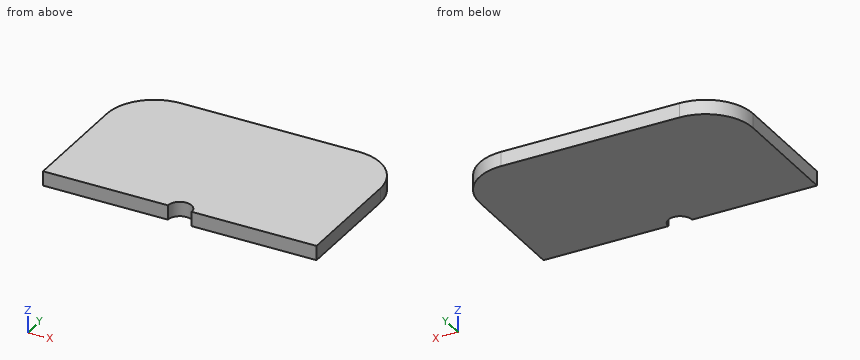
```python
from build123d import *

# Parameters (mm, degrees)
PAD_DEPTH = 15.45


with BuildPart() as part:
    # Sketch → Pad (new body)
    with BuildSketch(Plane.XY):
        with BuildLine():
            Line((-146.05, 36.5125), (-146.05, -87.3125))
            Line((-146.05, -87.3125), (-12.7, -87.3125))
            ThreePointArc((12.7, -87.3125), (0, -74.61), (-12.7, -87.3125))
            Line((12.7, -87.3125), (146.05, -87.3075))
            Line((146.05, -87.3075), (146.05, 36.5125))
            ThreePointArc((146.05, 36.5125), (131.171024, 72.433524), (95.25, 87.3125))
            Line((95.25, 87.3125), (-95.25, 87.3125))
            ThreePointArc((-95.25, 87.3125), (-131.171024, 72.433524), (-146.05, 36.5125))
        make_face()
    extrude(amount=PAD_DEPTH)


solid = part.part
```
Design review of the part built by this model. Coordinates are the model's own, in mm. Coordinates: 2 decimals unless noted, no trailing zeros. Loops run counter-clockwise (first coordinate to the right, second up) from the corner with the lowest first, then second, coordinate; pieces in that order, holes last. Notation, with made-up numbers: (26.25, 8.25) - (60.25, 8.25) arc R31 ccw to (60.25, 44.25) - close; hole circle Ø2 at (-33, 16). An arc over 180 degrees is marked (long way). Use CSV: the item, a comma, the result in double quotes. Start each with the question number.
1) Wall thickness on L1, parallel to Y at x = 57, z = 7; L2, parallel to X at y = -76, z = 9.25; L3, parallel to X at y = 64.5, z = 3.5: over which ranges is each line inside the solid? List them lowest first. Write a range as from..to.
2) Consider section A-A on z = 11.5. Write out the cut boundary in (x, y), then the cut area to 3 significant figures.
3) For pin 1 Ø5 at (y, z) = (48.5, 13) entering from +X, flat-tipped, find the tip position at first contact; note if it passes through.
4) Consider section B-B on x = 0. Write out the cut boundary in (y, z).
5) Consider section C-C on x = -125. Write out the cut boundary in (y, z), then the cut area to 3 significant figures.
Geometry says:
1,L1,"-87.31..87.31"
1,L2,"-146.05..-5.78, 5.78..146.05"
1,L3,"-137.65..137.65"
2,outline,"(-146.05, -87.31) - (-12.7, -87.31) arc R12.7 cw to (12.7, -87.31) - (146.05, -87.31) - (146.05, 36.51) arc R50.8 ccw to (95.25, 87.31) - (-95.25, 87.31) arc R50.8 ccw to (-146.05, 36.51) - close"
2,area,"49,600 mm^2"
3,pin 1,"x = 145.16"
4,outline,"(-74.61, 0) - (87.31, 0) - (87.31, 15.45) - (-74.61, 15.45) - close"
5,outline,"(-87.31, 0) - (77.69, 0) - (77.69, 15.45) - (-87.31, 15.45) - close"
5,area,"2,550 mm^2"
